Could you check a few things on this model? Use its own coordinates, in mm. Coordinates: 2 decimals unless noted, no trailing zeros. Order: outer loops, then holes, each group sorted by start corner. A loop starts at its lowest first (then second) coordinate and runs counter-clockwise, first axis right, second up. Notation, with made-up numbers: (45.25, -28.5) -> (63.25, -28.5) arc R5 cw to (63.25, -21.5) -> close; hole circle Ø1 at (54, -6.5). An arc over 180 degrees is marked (long way). Put each result on its own line as item: value. Start each with the question number.
Q1. Please list where these lines run through material, in increasing order: line 1 along X through (y, z) = (23.5, 9.25); line 2 along Y through (x, z) = (-42, 23); line 3 along Z through (x, y) = (-343, 24.25).
Q2. Will these pins go through, and if not, where does the flat tip stop? pin 1 (1.8 mm diameter, centred on x = -343, z = 9.5, fed in from +Y); pin 2 (3 mm diameter, centred on x = -104.5, y = 11, fed in from +Z).
Q3. If we section it at C-C (y = -15): Please give me the cut outline in (x, z).
Q4. If we section it at B-B (x = -262.5): Please give me the cut outline in (y, z), and give its area (4 significant figures).
Q5. If we section it at A-A (z = 20): Please give me the cut outline in (x, y).
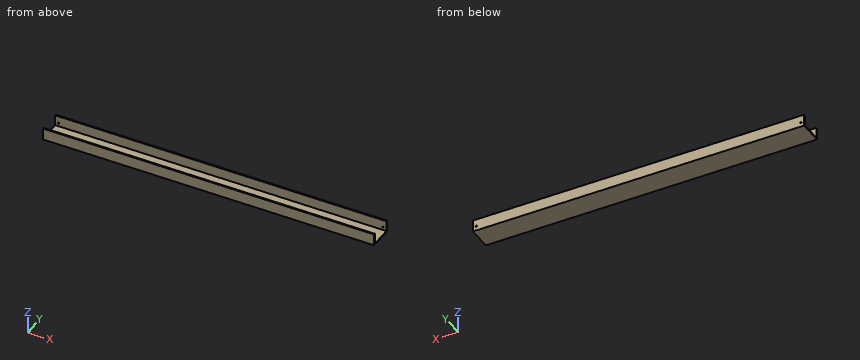
from build123d import *

# Parameters (mm, degrees)
F1_DEPTH      = 350
F1_DEPTH_BACK = 350
F3_D          = 3
F3_DEPTH      = 10


with BuildPart() as f1:
    # F0 (on Right) → F1 (new body, two sides)
    with BuildSketch(Plane.YZ) as f1_sk:
        Polygon((-25, 0), (25, 0), (25, 25), (22.5, 25), (22.5, 2.5), (-22.5, 2.5), (-22.5, 25), (-25, 25), align=None)
    extrude(amount=F1_DEPTH)
    extrude(f1_sk.sketch, amount=-F1_DEPTH_BACK)

    # F3
    with Locations(Plane.XZ.offset(-22.5)):
        with Locations((-343, 9.5), (343, 9.5)):
            Hole(F3_D / 2, depth=F3_DEPTH)


solid = f1.part
The answers:
1. line 1: -350 to -344.48, -341.52 to 341.52, 344.48 to 350
1. line 2: -25 to -22.5, 22.5 to 25
1. line 3: 0 to 8, 11 to 25
2. pin 1: y = -22.5
2. pin 2: z = 2.5
3. outline: (-350, 0) -> (350, 0) -> (350, 2.5) -> (-350, 2.5) -> close
4. outline: (-25, 0) -> (25, 0) -> (25, 25) -> (22.5, 25) -> (22.5, 2.5) -> (-22.5, 2.5) -> (-22.5, 25) -> (-25, 25) -> close
4. area: 237.5 mm^2
5. outline: (-350, -25) -> (350, -25) -> (350, -22.5) -> (-350, -22.5) -> close; (-350, 22.5) -> (350, 22.5) -> (350, 25) -> (-350, 25) -> close
